Check sheet for the drawn part. Datum: minimum x, y, z corner. Units: mm. Give positions to 0.01 mm unless a question says otherwise; leave off trailing zeros. Order: outer loops, then holes, each group sorted by start corner. A loop starts at its lowest first (then second) coordinate and runs counter-clockwise, first axis right, second up. Notation, with made-up numbers: (0.25, 26.25) - (44.25, 26.25) arc R36 ccw to (44.25, 61.25) - close; hole circle Ø1 at (71, -17.5). An arc over 180 degrees is marked (long way). Answer as a JSON object with one key per item and string values. Group by question number.
(1) Section check B-B (x = 2.5). Record the boundary of the cut face in (y, z).
(2) Section check C-C (y = 2.35). Count the separate pieces of the cut face and the enclosed holes in it, then the cut area to 3 significant figures.
(3) Depth check by flat-ended pin: pin 1 Ø12 at (x, z) = (12.5, 16) entering from -Y; pin 2 Ø0.9 at (y, z) = (2, 30.5) entering from -X; pin 3 Ø1.5 at (x, y) = (2, 2) entering from -Z. Enter the tip coordinate at first touch or a pass-through.
(4) Section check D-D (z = 21). Record the boundary of the cut face in (x, y) (3 decimals), then the cut area to 4 significant figures.
(5) Thickness scan on line 1 (Z direction, x = 12.5, y = 2.2); line 2 (X direction, y = 1.4, z = 21) (3 decimals); line 3 (Z direction, x = 30, y = 2.7). Record the ranges inside material, lowest first.
(6) Section check A-A (z = 35). Record the boundary of the cut face in (x, y) (3 decimals), then the cut area to 4 significant figures.
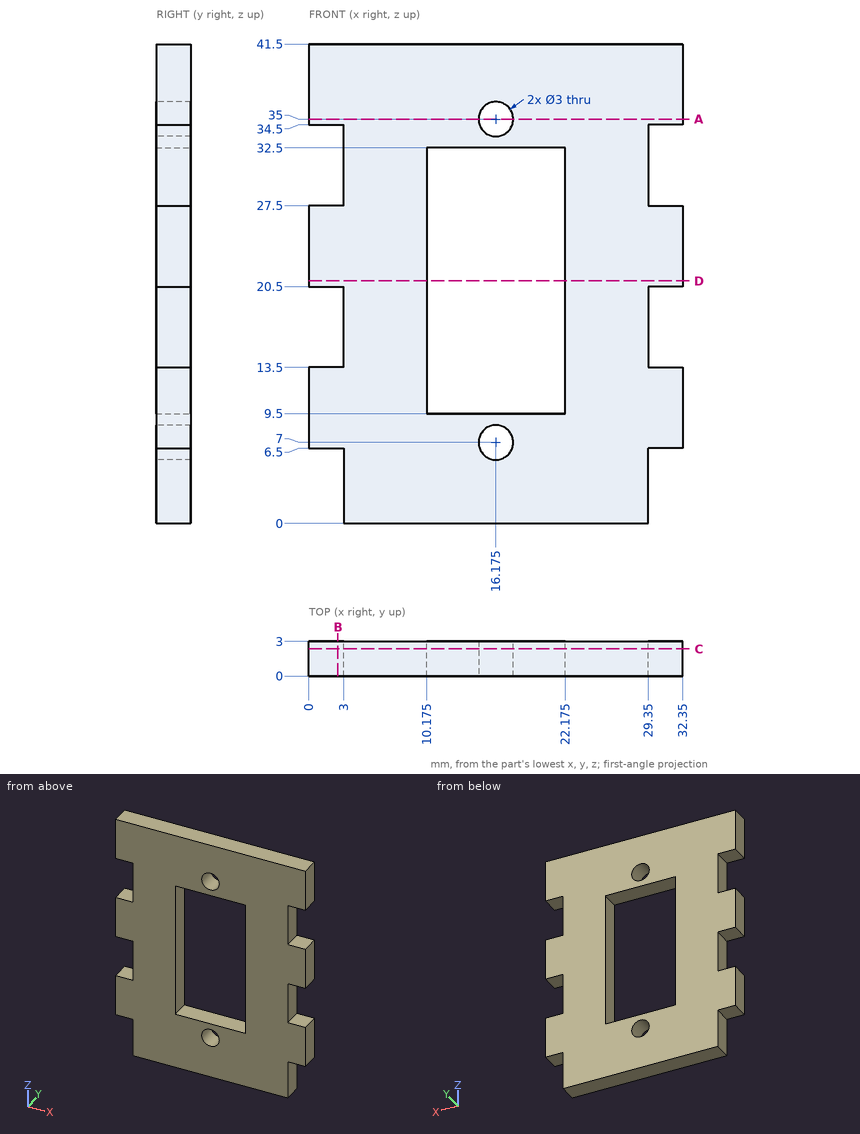
Solutions:
{
 "1": {"outline": "(0, 6.5) - (3, 6.5) - (3, 13.5) - (0, 13.5) - close; (0, 20.5) - (3, 20.5) - (3, 27.5) - (0, 27.5) - close; (0, 34.5) - (3, 34.5) - (3, 41.5) - (0, 41.5) - close"},
 "2": {"separate pieces": "1", "enclosed holes": "3", "area": "929 mm2"},
 "3": {"pin 1": "stops at y = 0", "pin 2": "stops at x = 3", "pin 3": "stops at z = 6.5"},
 "4": {"outline": "(0, 0) - (10.175, 0) - (10.175, 3) - (0, 3) - close; (22.175, 0) - (32.35, 0) - (32.35, 3) - (22.175, 3) - close", "area": "61.05 mm2"},
 "5": {"line 1": "z = 0 to 9.5, 32.5 to 41.5", "line 2": "x = 0 to 10.175, 22.175 to 32.35", "line 3": "z = 6.5 to 13.5, 20.5 to 27.5, 34.5 to 41.5"},
 "6": {"outline": "(0, 0) - (14.675, 0) - (14.675, 3) - (0, 3) - close; (17.675, 0) - (32.35, 0) - (32.35, 3) - (17.675, 3) - close", "area": "88.05 mm2"}
}
